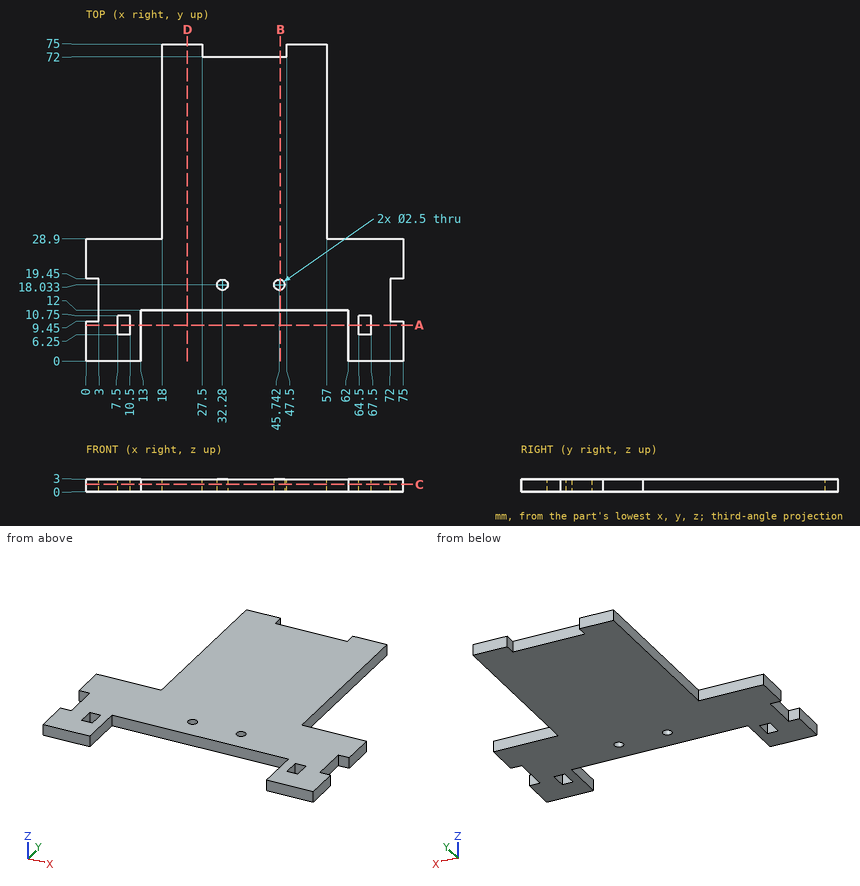
The figure shows three views and two pictorial views of one solid part (mm, origin at its lowest corner). Answer the questions. Give positions to 0.01 mm unless a question says otherwise; leave off trailing zeros. Write each loop counter-clockwise with the first axis right and the second up, starting at its lowest first coordinate (ties: lowest second). Pieces come first, ordered by that corner, then holes. Notation, with made-up numbers: (0.5, 23.5) -> (30.5, 23.5) arc R16 ccw to (30.5, 49.5) -> close; hole circle Ø2 at (-26.5, 15). An arc over 180 degrees is marked (long way). Answer as a JSON object with one key per item and string values.
1) Section C-C on z = 1.75 is taken. Count the separate pieces of the cut face and the enclosed holes in it, then the cut area to 3 significant figures.
Findings below:
{"separate pieces": "1", "enclosed holes": "4", "area": "3,220 mm^2"}
2) Section D-D on x = 24 is taken. Write down the section's boundary in (y, z), then the cut area to 3 significant figures.
Findings below:
{"outline": "(12, 0) -> (75, 0) -> (75, 3) -> (12, 3) -> close", "area": "189 mm^2"}
3) Section B-B on x = 46 is taken. Write down the section's boundary in (y, z).
Findings below:
{"outline": "(12, 0) -> (16.81, 0) -> (16.81, 3) -> (12, 3) -> close; (19.26, 0) -> (72, 0) -> (72, 3) -> (19.26, 3) -> close"}
4) Section A-A on y = 8.5 is taken. Write down the section's boundary in (x, z).
Findings below:
{"outline": "(0, 0) -> (7.5, 0) -> (7.5, 3) -> (0, 3) -> close; (10.5, 0) -> (13, 0) -> (13, 3) -> (10.5, 3) -> close; (62, 0) -> (64.5, 0) -> (64.5, 3) -> (62, 3) -> close; (67.5, 0) -> (75, 0) -> (75, 3) -> (67.5, 3) -> close"}
5) Flat-ended cylindrical pins translate along their axes: pin 1 Ø1 at (y, z) = (42, 1) entering from -X; pin 2 Ø0.9 at (x, z) = (8.5, 1.5) entering from +Y; pin 3 Ø1.5 at (y, z) = (74, 1) entering from +X; pin 4 Ø1 at (x, y) = (14, 29.5) entering from -Z. Find the tip coordinate at first contact, or state that the pin passes through.
Findings below:
{"pin 1": "stops at x = 18", "pin 2": "stops at y = 28.9", "pin 3": "stops at x = 57", "pin 4": "passes through"}
6) Straight lines are drawn through the part: probe 1 along X at (y, z) = (18, 2.85); probe 2 along X at (y, z) = (70, 1.35); probe 3 along Y at (x, z) = (24, 2.3). For each, find the intervals that lie inside material, in ascending order. Write a range as from..to.
Findings below:
{"probe 1": "x = 3..31.03, 33.53..44.49, 46.99..72", "probe 2": "x = 18..57", "probe 3": "y = 12..75"}
